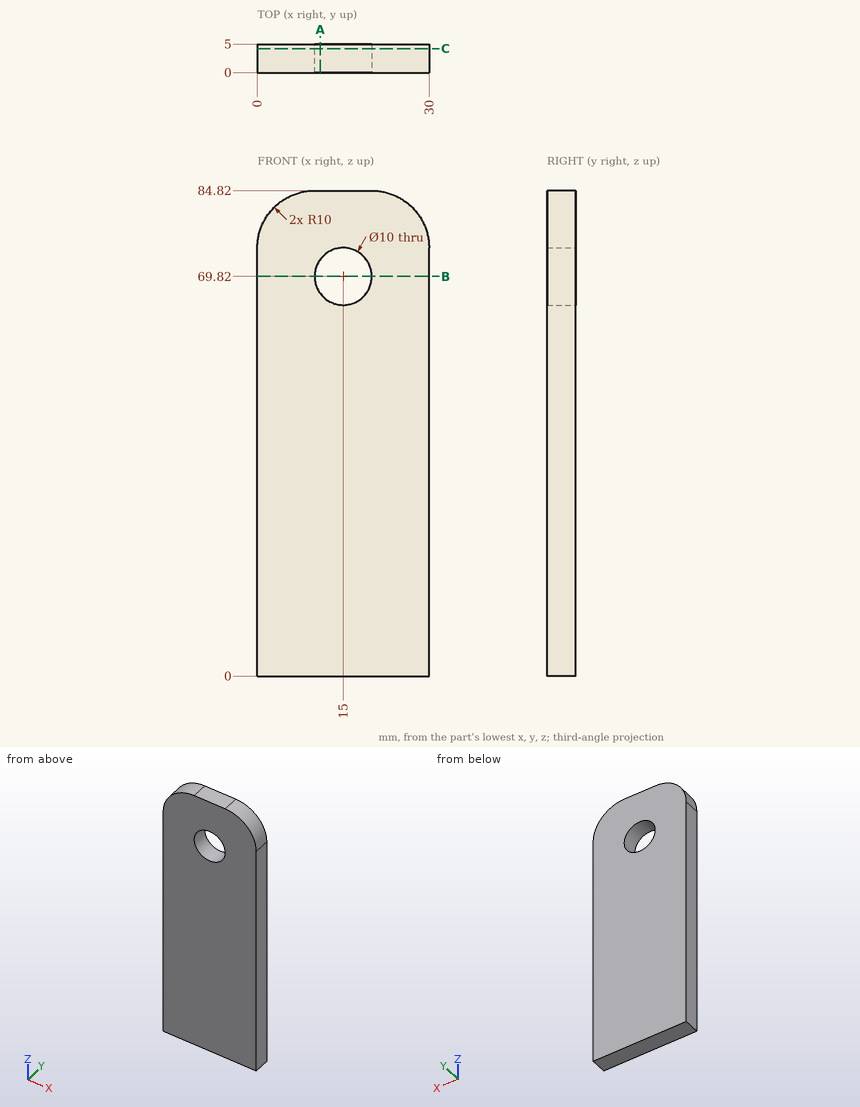
Here's the drawing with two shaded views (mm, measured from the low corner). I have some questions. Round coordinates to 2 decimals unless told otherwise and drop trailing zeros. Loops run counter-clockwise (first coordinate to the right, second up) from the corner with the lowest first, then second, coordinate; pieces in that order, holes last.
Item 1: Please list where these lines run through material, in increasing order: L1, parallel to Z at x = 15, y = 3.4; L2, parallel to Z at x = 9.5, y = 0.75; L3, parallel to Z at x = 16.5, y = 2.
Item 2: Suppose I cut it at C-C, the plane y = 4.2. Write out the boundary of the cut face in (x, z), then the cut area to 3 significant figures.
Item 3: Suppose I cut it at B-B, the plane z = 69.82. Write out the boundary of the cut face in (x, y), then the cut area to 3 significant figures.
Item 4: Suppose I cut it at A-A, the plane x = 11. Write out the boundary of the cut face in (y, z).
Reported:
1. L1: z = 0 to 64.82, 74.82 to 84.82
1. L2: z = 0 to 84.81
1. L3: z = 0 to 65.05, 74.59 to 84.82
2. outline: (0, 0) - (30, 0) - (30, 74.82) arc R10 ccw to (20, 84.82) - (10, 84.82) arc R10 ccw to (0, 74.82) - close; hole circle Ø10 at (15, 69.82)
2. area: 2,420 mm2
3. outline: (0, 0) - (10, 0) - (10, 5) - (0, 5) - close; (20, 0) - (30, 0) - (30, 5) - (20, 5) - close
3. area: 100 mm2
4. outline: (0, 0) - (5, 0) - (5, 66.82) - (0, 66.82) - close; (0, 72.82) - (5, 72.82) - (5, 84.82) - (0, 84.82) - close
